Source: three-view drawing plus pictorial views. Frame: mm from the lowest corner of the part. A direction names the side the tool comes from. Coordinates: 2 decimals unless noted, no trailing zeros. Write each loop counter-clockwise with the first axis right and the second up, starting at its lowest first coordinate (ties: lowest second). Pieces come first, ordered by that corner, then holes. Notation, with made-up numbers: (20.25, -2) - (30.25, -2) arc R8 cw to (30.25, 11) - close; hole circle Ø3 at (82.5, 82). An arc over 180 degrees is marked (long way). Answer as a JSON object with one key per item and string values. Group by question number.
Item 1: Section C-C on z = 12.75. Return loops of the section in (x, y).
Item 2: Set-up query: the marked faces 1, 2 and 3. Return all of +Z, -Z, +X, -X, +Y, -Y with unobstructed straight access to the full face (end or side cutting, diameter ignored); none if empty.
Item 3: Section B-B on x = 32. Return loops of the section in (y, z).
Item 4: Line query: line 1 along Y through (x, z) = (28.5, 2.75). Output: solid intervals per line, ascending. Write a range as from..to.
Item 5: Section A-A on z = 5.5. Return loops of the section in (x, y).
Item 6: First-contact query: pin 1 Ø0.9 at (y, z) = (1.5, 6) entering from -X; pin 2 Ø2.5 at (x, y) = (1.5, 26) entering from -Z; pin 3 Ø6 at (y, z) = (20.5, 15) entering from +X. Flat tips, straight axial feed; report the tip coordinate or a pass-through.
Item 7: Section D-D on y = 10.5. Return loops of the section in (x, z), and give its area (3 significant figures).
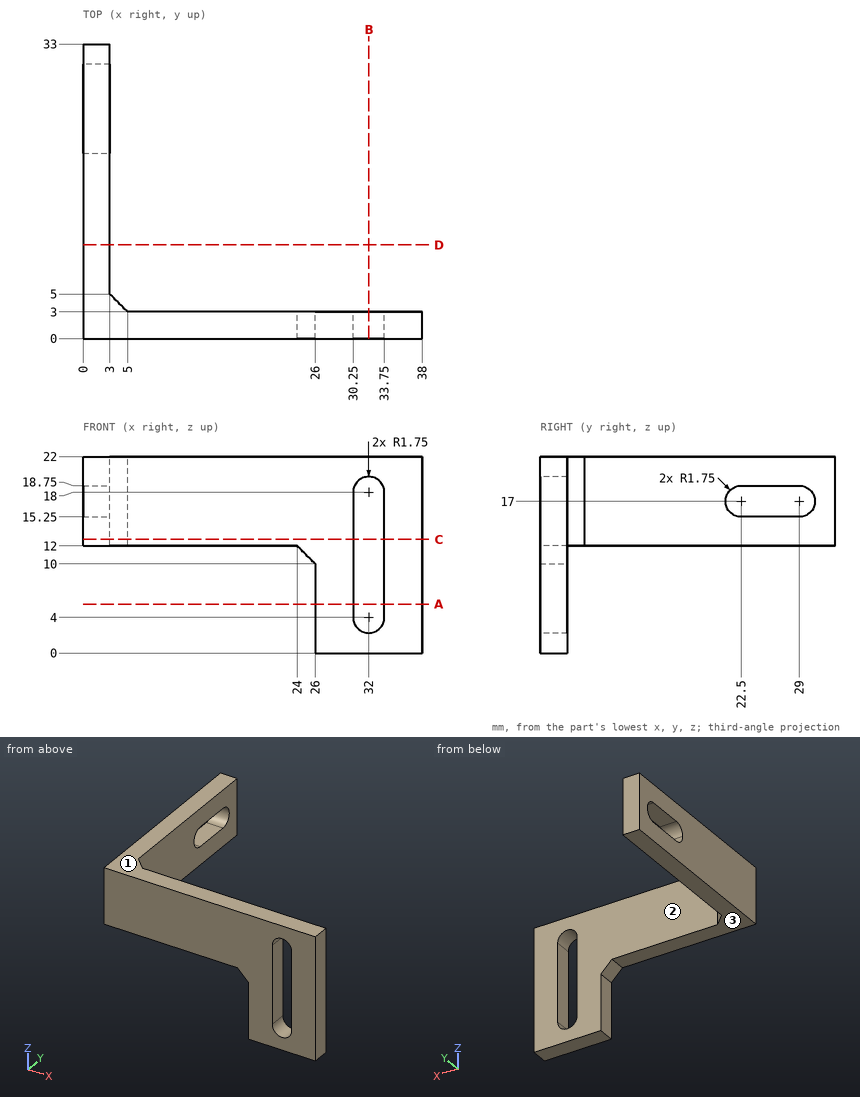
Checks:
{
 "1": {"outline": "(0, 0) - (30.25, 0) - (30.25, 3) - (5, 3) - (3, 5) - (3, 33) - (0, 33) - close; (33.75, 0) - (38, 0) - (38, 3) - (33.75, 3) - close"},
 "2": {"face 1": "+Z, +X, -X, +Y, -Y", "face 2": "+Z, -Z, +X, +Y", "face 3": "-Z, -X, +Y, -Y"},
 "3": {"outline": "(0, 0) - (3, 0) - (3, 2.25) - (0, 2.25) - close; (0, 19.75) - (3, 19.75) - (3, 22) - (0, 22) - close"},
 "4": {"line 1": "0..3"},
 "5": {"outline": "(26, 0) - (30.25, 0) - (30.25, 3) - (26, 3) - close; (33.75, 0) - (38, 0) - (38, 3) - (33.75, 3) - close"},
 "6": {"pin 1": "x = 26", "pin 2": "z = 12", "pin 3": "x = 3"},
 "7": {"outline": "(0, 12) - (3, 12) - (3, 22) - (0, 22) - close", "area": "30.0 mm^2"}
}
